Work out the finished part from the listing and answer in its coordinate system (mm). Round coordinates to 2 decimals unless told otherwise and drop trailing zeros. Write each loop counter-clockwise with the first axis right and the second up, starting at its lowest first coordinate (ties: lowest second). Pieces come first, ordered by that corner, then holes. Notation, with made-up numbers: M -10.5,24 L 28.5,24 A27 cw 28.5,52 Z; hole C 51,52.25 d1. An arc over 180 degrees is marked long. One line per item, written item: value. Start each with the question number.
Q1. Given pin 1 Ø1.5 at (x, y) = (470.5, -377) entering from -Z, flat-ended and moving along its own axis, determine where the tip first touches the part or whether it passes through.
Q2. Find section A-A (y = -374). Write down the section's boundary in (x, z) (3 decimals).
Q3. Consider probe 1 along X at (y, z) = (-373, 2.5) (3 decimals); probe 2 along X at (y, z) = (-289, 11.5); probe 3 along Z at (x, y) = (189, -90.5). Determine where each line is inside the solid, lowest interval first.
from build123d import *

# Parameters (mm, degrees)
SKETCH1_W           = 560.57
SKETCH1_H           = 482.6
BOSS_EXTRUDE1_DEPTH = 44.45
CUT_EXTRUDE1_DEPTH  = 152.4


with BuildPart() as part:
    # Sketch1 → Boss-Extrude1 (new body)
    with BuildSketch(Plane.XY):
        with Locations((280.285, -241.3)):
            Rectangle(SKETCH1_W, SKETCH1_H)
    extrude(amount=BOSS_EXTRUDE1_DEPTH)

    # Sketch2 → Cut-Extrude1 (cut, symmetric)
    with BuildSketch(Plane(origin=(0, -241.3, 0), x_dir=(-1, 0, 0), z_dir=(0, -1, 0))):
        with BuildLine():
            Line((-485.135, 0), (-485.135, -10))
            ThreePointArc((-485.135, -10), (-467.07, -23.003655986), (-449.005, -10))
            Line((-449.005, -10), (-449.005, 0))
            Line((-449.005, 0), (-485.135, 0))
        make_face()
        with BuildLine():
            Line((-391.635, -10), (-391.635, 0))
            Line((-391.635, 0), (-355.505, 0))
            Line((-355.505, 0), (-355.505, -10))
            ThreePointArc((-355.505, -10), (-373.57, -23.003655986), (-391.635, -10))
        make_face()
    cut_extrude1 = extrude(amount=CUT_EXTRUDE1_DEPTH, both=True, mode=Mode.SUBTRACT)

    # Mirror1: Cut-Extrude1 across plane
    add(cut_extrude1.mirror(Plane.ZY.offset(-280.285)), mode=Mode.SUBTRACT)


solid = part.part
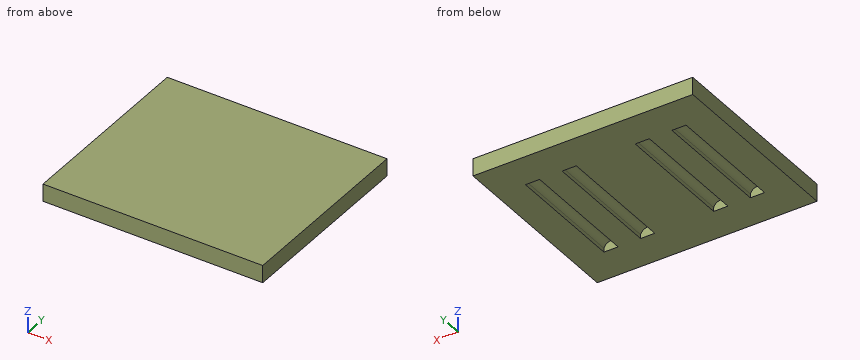
The answers:
1. pin 1: z = 22.54
2. outline: M 0,0 L 75.435,0 L 75.435,10 A19.05 cw 111.565,10 L 111.565,0 L 168.935,0 L 168.935,10 A19.05 cw 205.065,10 L 205.065,0 L 355.505,0 L 355.505,10 A19.05 cw 391.635,10 L 391.635,0 L 449.005,0 L 449.005,10 A19.05 cw 485.135,10 L 485.135,0 L 560.57,0 L 560.57,44.45 L 0,44.45 Z
3. probe 1: 0 to 75.435, 111.565 to 168.935, 205.065 to 355.505, 391.635 to 449.005, 485.135 to 560.57
3. probe 2: 0 to 76.01, 110.99 to 169.51, 204.49 to 356.08, 391.06 to 449.58, 484.56 to 560.57
3. probe 3: 22.9 to 44.45
